CAD build for the part. Positions are in the model's coordinates, mm. Face numbers are marked on the shaded views. A direction names the side the tool comes from. Give positions to 0.01 mm unless a question says otherwise; leave off trailing zeros. Write each loop counter-clockwise with the first axis right and the second up, starting at its lowest first coordinate (ties: lowest second). Pieces come first, ordered by that corner, then holes. Notation, with made-up numbers: (83.5, 41) - (140.5, 41) arc R12 cw to (140.5, 59) - close; hole circle Ø10 at (46.25, 39.5). An arc over 180 degrees is marked (long way). Write item = value, one per line. Start each with the question number.
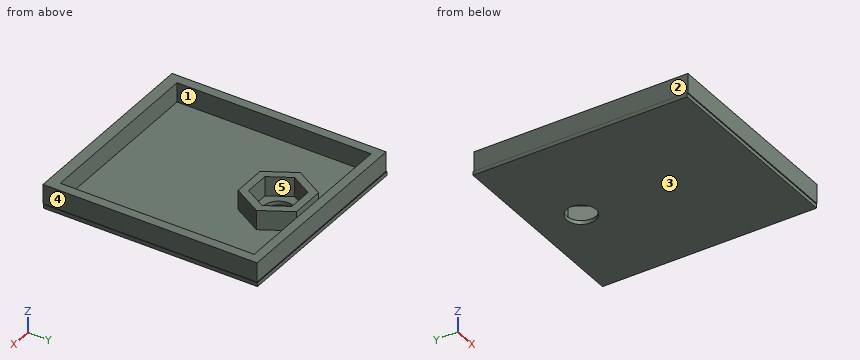
```python
from build123d import *

# Parameters (mm, degrees)
PAD005_DEPTH  = 5
SKETCH007_W   = 50.955005
SKETCH007_H   = 55
SKETCH007_R   = 3.75
PAD006_DEPTH  = 1
SKETCH008_W   = 50.8
SKETCH008_H   = 55
SKETCH008_W_2 = 46
SKETCH008_H_2 = 49.832681
PAD007_DEPTH  = 5


with BuildPart() as part:
    # Sketch006 → Pad005 (new body)
    with BuildSketch(Plane.XY):
        Polygon((4.330127, 47.5), (8.660254, 55), (4.330127, 62.5), (-4.330127, 62.5), (-8.660254, 55), (-4.330127, 47.5), align=None)
        Polygon((3.204294, 49.45), (6.408588, 55), (3.204294, 60.55), (-3.204294, 60.55), (-6.408588, 55), (-3.204294, 49.45), align=None, mode=Mode.SUBTRACT)
    extrude(amount=PAD005_DEPTH)

    # Sketch007 → Pad006 (join)
    with BuildSketch(Plane.XY):
        with Locations((0.077502, 38.828427)):
            Rectangle(SKETCH007_W, SKETCH007_H)
        with Locations((0, 55.078962)):
            Circle(SKETCH007_R, mode=Mode.SUBTRACT)
    extrude(amount=-PAD006_DEPTH)

    # Sketch008 → Pad007 (join)
    with BuildSketch(Plane.XY):
        with Locations((0, 38.613518)):
            Rectangle(SKETCH008_W, SKETCH008_H)
        with Locations((0, 38.883774)):
            Rectangle(SKETCH008_W_2, SKETCH008_H_2, mode=Mode.SUBTRACT)
    extrude(amount=PAD007_DEPTH)


solid = part.part
```
1. Cut at D-D (x = -11.5). Give the cut face in (y, z), then the cut area to 3 significant figures.
2. Wall check: line 1 along Y through (x, z) = (-3, 3); line 2 along Y through (x, z) = (0, -0.4); line 3 along X through (y, z) = (17.5, 2.65). Give the ranges that are in metal, low to high.
3. Cut at B-B (z = 1.8). Give the cut face in (x, y), then the cut area to 3 significant figures.
4. Cut at C-C (y = 20). Give the cut face in (x, z) (3 decimals).
5. Tool access for the marked faces 4 and 5: list every direction of +Z, -Z, +X, -X, +Y, -Y with a clear straight run to the whole face (end or side of a thin tool).
6. Mould opens along X. For the marked faces 1, 2 and 3 say: +X half, -X half, draft (parallel to the pull), parting line (faces both ways), or undercut.
7. Pin check, flat tips, straight feed: pin 1 Ø1.5 at (x, z) = (6, 3) entering from +Y; pin 2 Ø0.8 at (x, z) = (-12, -0.5) entering from -Y; pin 3 Ø23 at (x, y) = (-2.5, 28.5) entering from +Z. Stop position of each tip, or through.
8. Cut at A-A (x = 0). Give the cut face in (y, z), then the cut area to 3 significant figures.
Output:
q1.outline = (11.11, 0) - (11.33, 0) - (11.33, -1) - (66.33, -1) - (66.33, 0) - (66.11, 0) - (66.11, 5) - (63.8, 5) - (63.8, 0) - (13.97, 0) - (13.97, 5) - (11.11, 5) - close
q1.area = 80.8 mm2
q2.line_1 = 11.11 to 13.97, 47.5 to 49.45, 60.55 to 62.5, 63.8 to 66.11
q2.line_2 = 11.33 to 51.33, 58.83 to 66.33
q2.line_3 = -25.4 to -23, 23 to 25.4
q3.outline = (-25.4, 11.11) - (25.4, 11.11) - (25.4, 66.11) - (-25.4, 66.11) - close; (-8.66, 55) - (-4.33, 47.5) - (4.33, 47.5) - (8.66, 55) - (4.33, 62.5) - (-4.33, 62.5) - close; hole (-23, 13.97) - (23, 13.97) - (23, 63.8) - (-23, 63.8) - close; hole (-6.41, 55) - (-3.2, 49.45) - (3.2, 49.45) - (6.41, 55) - (3.2, 60.55) - (-3.2, 60.55) - close
q3.area = 590 mm2
q4.outline = (-25.4, -1) - (25.555, -1) - (25.555, 0) - (25.4, 0) - (25.4, 5) - (23, 5) - (23, 0) - (-23, 0) - (-23, 5) - (-25.4, 5) - close
q5.face_4 = +Z, +X, +Y, -Y
q5.face_5 = +Z
q6.face_1 = undercut
q6.face_2 = -X half
q6.face_3 = draft
q7.pin_1 = 66.11
q7.pin_2 = 11.33
q7.pin_3 = 0
q8.outline = (11.11, 0) - (11.33, 0) - (11.33, -1) - (51.33, -1) - (51.33, 0) - (49.45, 0) - (49.45, 5) - (47.5, 5) - (47.5, 0) - (13.97, 0) - (13.97, 5) - (11.11, 5) - close; (58.83, -1) - (66.33, -1) - (66.33, 0) - (66.11, 0) - (66.11, 5) - (63.8, 5) - (63.8, 0) - (62.5, 0) - (62.5, 5) - (60.55, 5) - (60.55, 0) - (58.83, 0) - close
q8.area = 92.8 mm2
